For this review, take the finished solid that the model builds, in its own axes (mm). Round coordinates to 2 decimals unless told otherwise and drop trailing zeros. Order: outer loops, then holes, each group sorted by start corner. A loop starts at its lowest first (then second) coordinate and runs counter-clockwise, first axis right, second up. Notation, with made-up numbers: M -26,6 L 30,6 A24 ccw 30,29 Z; hole C 17,-36 d4. An arc over 180 degrees is marked long. Use a Markdown table: item, result.
Autodesk Inventor part; units mm, degrees
ref_plane "YZ Plane" through (0, 0, 0) normal (1, 0, 0) x (0, 1, 0)
ref_plane "XZ Plane" through (0, 0, 0) normal (0, 1, 0) x (-1, 0, 0)
ref_plane "XY Plane" through (0, 0, 0) normal (0, 0, 1) x (1, 0, 0)
sketch "Sketch1" plane through (0, 0, 0) normal (0, 0, 1) x (1, 0, 0)
  circle A0 centre (0, 0) radius 17.5
  dimension "d0" = 35
extrude "Extrusion1" add sketch "Sketch1" along normal blind 45
sketch "Sketch2" plane through (0, 0, 45) normal (0, 0, 1) x (1, 0, 0)
  line L0 (12.5, 21.9531) -> (30.6636, 21.9531)
  line L1 (30.6636, 21.9531) -> (30.6636, -19.8764)
  line L2 (30.6636, -19.8764) -> (12.5, -19.8764)
  line L3 (12.5, -19.8764) -> (12.5, 21.9531)
  point P0 (0, 0)
  dimension "d3" = 12.5
extrude "Extrusion2" cut sketch "Sketch2" against normal through all
pattern_circular "Circular Pattern1" count 2 over 360 about axis through (0, 0, 0) along (0, 0, 1) of "Extrusion2"
sketch "Sketch3" plane through (12.5, -12.2474, 45) normal (1, 0, 0) x (0, 0, -1)
  circle A0 centre (29, 12.2474) radius 9
  line L0 (45, 24.4949) -> (45, 0)
  point P0 (45, 12.2474)
  point P1 (45, 12.2474)
  dimension "d9" = 18
  dimension "d10" = 16
extrude "Extrusion3" cut sketch "Sketch3" against normal through all
sketch "Sketch4" plane through (0, 0, 45) normal (0, 0, 1) x (1, 0, 0)
  arc A0 (12.5, 12.2474) -> (-12.5, 12.2474) centre (0, 0) ccw
hole "Hole1" at (0, 0, 45) direction (0, 0, -1) diameter 10.647 depth 25 tip angle 118
chamfer "Chamfer1" distance 4 angle 45 4 edges at (0, 17.5, 0) (0, -17.5, 0) (0, 17.5, 45) (0, -17.5, 45)
chamfer "Chamfer2" distance 1 angle 45 1 edges at (0, 5.3235, 45)
chamfer "Chamfer3" distance 1 angle 45 2 edges at (12.5, 0, 25) (-12.5, 0, 25)
properties part number "IMS-01-001" material "Steel, Carbon"
Q1. Add section A-A (y = 0). Write out the cut boundary in (x, z).
Determined:
| item | result |
|---|---|
| outline | M -12.5,0 L 12.5,0 L 12.5,6 L 11.5,7 L -11.5,7 L -12.5,6 Z; M -12.5,26 L -11.5,25 L -5.32,25 L -5.32,44 L -6.32,45 L -12.5,45 Z; M 5.32,25 L 11.5,25 L 12.5,26 L 12.5,45 L 6.32,45 L 5.32,44 Z |
Q2. Wall thickness on line 1 along X through (y, z) = (0, 28); line 2 along Y through (x, z) = (4, 16); line 3 along X through (y, z) = (12.5, 37): over which ranges is each line inside the solid? List them lowest first. Write a range as [from, to].
Determined:
| item | result |
|---|---|
| line 1 | x = [-12.5, -5.32], [5.32, 12.5] |
| line 2 | y = [-17.04, -9], [9, 17.04] |
| line 3 | x = [-12.25, 12.25] |
Q3. Add section B-B (z = 16). Write out the cut boundary in (x, y), then the cut area to 3 significant figures.
Determined:
| item | result |
|---|---|
| outline | M -12.5,-12.25 A17.5 ccw 12.5,-12.25 L 12.5,-10 L 11.5,-9 L -11.5,-9 L -12.5,-10 Z; M -12.5,10 L -11.5,9 L 11.5,9 L 12.5,10 L 12.5,12.25 A17.5 ccw -12.5,12.25 Z |
| area | 341 mm^2 |
Q4. Draft analysis for pull direction X (two halves, no side actions). For faces 1 (the flat face through (-12.5, 0, 28)), 2 (the cylindrical face through (-0.23, 5.32, 33.48)), 3 (the conical face through (0.2, -14.2, 44.3)), state which applies: pulls with the +X half, pulls with the -X half, needs draft (parallel to the pull), parting line crosses it, or undercut.
Determined:
| item | result |
|---|---|
| face 1 | pulls with the -X half |
| face 2 | undercut |
| face 3 | parting line crosses it |
Q5. Add section C-C (x = 0). Write out the cut boundary in (y, z), then the cut area to 3 significant figures.
Determined:
| item | result |
|---|---|
| outline | M -17.5,4 L -13.5,0 L 13.5,0 L 17.5,4 L 17.5,41 L 13.5,45 L 6.32,45 L 5.32,44 L 5.32,23.26 A9 cw long -5.32,23.26 L -5.32,44 L -6.32,45 L -13.5,45 L -17.5,41 Z |
| area | 1,070 mm^2 |
Q6. Add section D-D (z = 36). Write out the cut boundary in (x, y), then the cut area to 3 significant figures.
Determined:
| item | result |
|---|---|
| outline | M -12.5,-12.25 A17.5 ccw 12.5,-12.25 L 12.5,12.25 A17.5 ccw -12.5,12.25 Z; hole C 0,0 d10.65 |
| area | 704 mm^2 |
Q7. Clearance check with flat-ended pins moving along their axes: pin 1 (6.5 mm diameter, centred on x = 0, y = 0, fed in from -Z); pin 2 (1 mm diameter, centred on x = -7, z = 11.5, fed in from -Y); pin 3 (12 mm diameter, centred on x = -9.5, z = 40, fed in from -Y); pin 4 (2 mm diameter, centred on x = -4, z = 8.5, fed in from -Y). State where each tip first meets the part, or that it passes through.
Determined:
| item | result |
|---|---|
| pin 1 | stops at z = 0 |
| pin 2 | stops at y = -16.25 |
| pin 3 | stops at y = -17.15 |
| pin 4 | stops at y = -17.24 |
